from build123d import *

# Parameters (mm, degrees)
F0_W     = 50
F0_H     = 14
F1_DEPTH = 10
F2_D     = 8.5


with BuildPart() as f1:
    # F0 (on Right) → F1 (new body)
    with BuildSketch(Plane.YZ):
        with Locations((-25.7008373737, 14.168410562)):
            Rectangle(F0_W, F0_H)
    extrude(amount=F1_DEPTH)

    # F2 (through all)
    with Locations(Plane(origin=(0, 0, 0), x_dir=(0, 1, 0), z_dir=(-1, 0, 0))):
        with Locations((-40.7008373737, -14.168410562), (-10.7008373737, -14.168410562)):
            Hole(F2_D / 2)


solid = f1.part
Part model, mm, in its own coordinate system. Give positions to 0.01 mm unless a question says otherwise; leave off trailing zeros. Write each loop counter-clockwise with the first axis right and the second up, starting at its lowest first coordinate (ties: lowest second). Pieces come first, ordered by that corner, then holes.
1) Cut at C-C on z = 13. Write the cut outline in (x, y), then the cut area to 3 significant figures.
Resolved:
outline: (0, -50.7) - (10, -50.7) - (10, -44.79) - (0, -44.79) - close; (0, -36.61) - (10, -36.61) - (10, -14.79) - (0, -14.79) - close; (0, -6.61) - (10, -6.61) - (10, -0.7) - (0, -0.7) - close
area: 337 mm2
2) Cut at A-A on z = 10.5. Write the cut outline in (x, y), then the cut area to 3 significant figures.
Resolved:
outline: (0, -50.7) - (10, -50.7) - (10, -42.85) - (0, -42.85) - close; (0, -38.55) - (10, -38.55) - (10, -12.85) - (0, -12.85) - close; (0, -8.55) - (10, -8.55) - (10, -0.7) - (0, -0.7) - close
area: 414 mm2
3) Cut at B-B on x = 1.5. Write the cut outline in (y, z), then the cut area to 3 significant figures.
Resolved:
outline: (-50.7, 7.17) - (-0.7, 7.17) - (-0.7, 21.17) - (-50.7, 21.17) - close; hole circle Ø8.5 at (-40.7, 14.17); hole circle Ø8.5 at (-10.7, 14.17)
area: 587 mm2
4) Two-plate mould, pull along Z, no slides. Class faces 1 (the face through (5, -26, 21.168)), 2 (the face through (5.07, -44.755, 12.892)), 3 (the face through (5, -0.701, 14)), 4 (the face through (5, -26, 7.168)): released by +Z, released by -Z, zero draft, split by the parting line, or undercut.
Resolved:
face 1: released by +Z
face 2: undercut
face 3: zero draft
face 4: released by -Z
5) Probe L1, parallel to Y at x = 0.5, z = 11; L2, parallel to Y at x = 5.25, z = 15; L3, parallel to Z at x = 1.75, y = -38.5. List the from-to ranges inside material, lowest first.
Resolved:
L1: y = -50.7 to -43.53, -37.87 to -13.53, -7.87 to -0.7
L2: y = -50.7 to -44.87, -36.53 to -14.87, -6.53 to -0.7
L3: z = 7.17 to 10.53, 17.8 to 21.17
